from build123d import *

# Parameters (mm, degrees)
SKETCH1_R           = 9.5
SKETCH1_R_2         = 6.35
BOSS_EXTRUDE1_DEPTH = 13.25
SKETCH2_W           = 73.338944958
SKETCH2_H           = 12.5
CUT_EXTRUDE3_DEPTH  = 38


with BuildPart() as part:
    # Sketch1 → Boss-Extrude1 (new, symmetric)
    with BuildSketch(Plane(origin=(0, 0, 0), x_dir=(1, 0, 0), z_dir=(0, 1, 0))):
        with BuildLine():
            Line((0, 0), (-62, 0))
            ThreePointArc((-62, 0), (-75.125587601, 4.90964049), (-81.806983567, 17.228104986))
            Line((-81.806983567, 17.228104986), (-88.547021707, 65.390038979))
            ThreePointArc((-88.547021707, 65.390038979), (-78.78369233, 80.716074763), (-62.110282709, 73.49060696))
            ThreePointArc((-62.110282709, 73.49060696), (-36.56849942, 45.611382856), (0, 36))
            Line((0, 36), (0, 26.5))
            Line((0, 26.5), (-22, 26.5))
            ThreePointArc((-22, 26.5), (-28.5, 20), (-22, 13.5))
            Line((-22, 13.5), (0, 13.5))
            Line((0, 13.5), (0, 0))
        make_face()
        with Locations(Location((-62, 20, 0), (0, 0, 270))):
            Circle(SKETCH1_R, mode=Mode.SUBTRACT)
        with Locations(Location((-74.68213321, 67.330365488, 0), (0, 0, 270))):
            Circle(SKETCH1_R_2, mode=Mode.SUBTRACT)
    extrude(amount=BOSS_EXTRUDE1_DEPTH, both=True)

    # Sketch2 → Cut-Extrude3 (cut)
    with BuildSketch(Plane(origin=(0, 0, 0), x_dir=(0, 0, -1), z_dir=(1, 0, 0))):
        with Locations((36.669472479, 0)):
            Rectangle(SKETCH2_W, SKETCH2_H)
    extrude(amount=-CUT_EXTRUDE3_DEPTH, mode=Mode.SUBTRACT)


solid = part.part
Check sheet for the modelled part. Datum: model origin and axes. Units: mm. A direction names the side the tool comes from. Give positions to 0.01 mm unless a question says otherwise; leave off trailing zeros. Loops run counter-clockwise (first coordinate to the right, second up) from the corner with the lowest first, then second, coordinate; pieces in that order, holes last. Notation, with made-up numbers: M 74,-20 L 96,-20 A7 ccw 96,-11 Z; hole C 42,-33.5 d10. An arc over 180 degrees is marked long. Return JSON: item names as keys, results as strings. Group by question number.
1. Cross-section at C-C on y = 3.75. Record the boundary of the cut face in (x, z) (3 decimals).
2. Cross-section at A-A on z = -62.5. Record the boundary of the cut face in (x, y).
3. Tool access check on faces 1 (the flat face through (-23, -6.25, -13)), 2 (the flat face through (-54, -13.25, -32)), 3 (the flat face through (-11, -10, -13.5)). Record the directions out of +Z, -Z, +X, -X, +Y, -Y that give a thin tool (end or side, any length) a straight path to the whole face; none if there is none.
4. Go/stop test with flat-tipped pins: pin 1 (1.5 mm diameter, centred on y = 9, z = -66.5, fed in from +X); pin 2 (12 mm diameter, centred on y = 7, z = -61.5, fed in from +X); pin 3 (7.5 mm diameter, centred on x = -7.5, y = -8, fed in from -Z); pin 4 (7.5 mm diameter, centred on x = -8, y = 9.5, fed in from +Z). Record where each tip stops, or that it passes through.
5. Mould release check, pull along Z, two halves, no side actions. Record for faces 4 (the flat face through (0, -10, -7)), 5 (the flat face through (-11, 10, -13.5)), 6 (the cylindrical face through (-43.98, 0.19, -50.8)): released by +Z, released by -Z, zero draft, split by the parting line, or undercut.
6. Thickness scan on L1, parallel to Y at x = -28, z = -31.5; L2, parallel to X at y = 12.25, z = -71; L3, parallel to X at y = -7.75, z = -68. Record the ranges inside material, lowest first.
7. Cross-section at D-D on x = -31. Record the boundary of the cut face in (y, z), plus the area to 3 significant figures.
8. Cross-section at B-B on x = -19. Record the boundary of the cut face in (y, z), plus the area to 3 significant figures.
Return value:
{
 "1": {"outline": "M -88.547,-65.39 A14 ccw -62.11,-73.491 A67 cw -38,-46.5 L -38,0 L -62,0 A20 ccw -81.807,-17.228 Z; hole C -74.682,-67.33 d12.7; hole C -62,-20 d19"},
 "2": {"outline": "M -88.14,-13.25 L -78.8,-13.25 L -78.8,13.25 L -88.14,13.25 Z; M -70.56,-13.25 L -55.34,-13.25 L -55.34,13.25 L -70.56,13.25 Z"},
 "3": {"face 1": "+Z, -Z, +X", "face 2": "+Z, -Z, +X, -X, -Y", "face 3": "+X, +Y, -Y"},
 "4": {"pin 1": "x = -57.65", "pin 2": "x = -49.23", "pin 3": "z = -36.62", "pin 4": "z = 0"},
 "5": {"face 4": "zero draft", "face 5": "undercut", "face 6": "released by -Z"},
 "6": {"L1": "-13.25 to -6.25, 6.25 to 13.25", "L2": "-88.19 to -79.86, -69.5 to -60.82", "L3": "-88.67 to -81, -68.37 to -59.09"},
 "7": {"outline": "M -13.25,-42.6 L -6.25,-42.6 L -6.25,0 L -13.25,0 Z; M 6.25,-42.6 L 13.25,-42.6 L 13.25,0 L 6.25,0 Z", "area": "596 mm^2"},
 "8": {"outline": "M -13.25,-38.18 L -6.25,-38.18 L -6.25,-26.5 L -13.25,-26.5 Z; M -13.25,-13.5 L -6.25,-13.5 L -6.25,0 L -13.25,0 Z; M 6.25,-38.18 L 13.25,-38.18 L 13.25,-26.5 L 6.25,-26.5 Z; M 6.25,-13.5 L 13.25,-13.5 L 13.25,0 L 6.25,0 Z", "area": "353 mm^2"}
}
